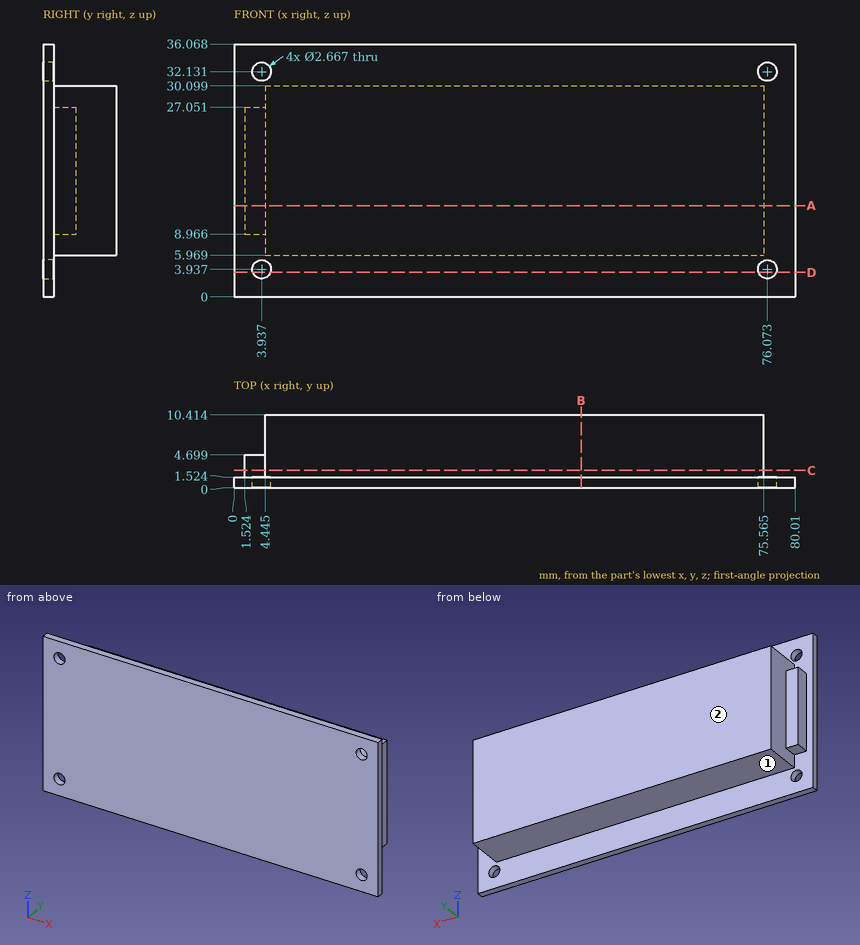
Here's the drawing with two shaded views (mm, measured from the low corner). I have some questions. A direction names the side the tool comes from. Coordinates: 2 decimals unless noted, no trailing zeros. Order: outer loops, then holes, each group sorted by start corner. A loop starts at its lowest first (then second) coordinate and runs counter-clockwise, first axis right, second up. Notation, with made-up numbers: (26, 35.25) - (76, 35.25) arc R17 ccw to (76, 50.25) - close; hole circle Ø8 at (-25.75, -32). An arc over 180 degrees is marked (long way). Answer in a Markdown table with one row per item. Add a question column.
(1) If we section it at B-B, the plane x = 49.5: Please give me the cut outline in (y, z).
(2) If we section it at A-A, the plane z = 13: Please give me the cut outline in (x, y) (3 decimals).
(3) If we section it at C-C, the plane y = 2.5: Please give me the cut outline in (x, z) (1 decimal), then the cut area to 3 significant figures.
(4) On a 3-axis mill with a long thin cutter (end or side, diameter ignored), from which of +Z, -Z, +X, -X, +Y, -Y can I reach the whole of each face in a straight line? I mean the marked faces 1 and 2. Say none if no direction works.
(5) If we section it at D-D, the plane z = 3.5: Please give me the cut outline in (x, y).
(6) Will these pins go through, and if not, where does the flat tip stop? pin 1 (3 mm diameter, centred on x = 26.5, y = 3.5, fed in from -Z); pin 2 (1.6 mm diameter, centred on y = 4, z = 16.5, fed in from -X); pin 3 (2.5 mm diameter, centred on x = 2.5, y = 4, fed in from -Z).
(7) I need wall thicknesses on L1, parallel to Y at x = 8, z = 35.5; L2, parallel to Z at x = 27.5, y = 4.5; L3, parallel to X at y = 6, z = 18.5 (3 decimals). Which ranges of each line are inside material? Lowest first, please.
Results are:
| question | item | result |
|---|---|---|
| 1 | outline | (0, 0) - (1.52, 0) - (1.52, 5.97) - (10.41, 5.97) - (10.41, 30.1) - (1.52, 30.1) - (1.52, 36.07) - (0, 36.07) - close |
| 2 | outline | (0, 0) - (80.01, 0) - (80.01, 1.524) - (75.565, 1.524) - (75.565, 10.414) - (4.445, 10.414) - (4.445, 4.699) - (1.524, 4.699) - (1.524, 1.524) - (0, 1.524) - close |
| 3 | outline | (1.5, 9) - (4.4, 9) - (4.4, 6) - (75.6, 6) - (75.6, 30.1) - (4.4, 30.1) - (4.4, 27.1) - (1.5, 27.1) - close |
| 3 | area | 1,770 mm2 |
| 4 | face 1 | -Z, +X, -X, +Y |
| 4 | face 2 | +Z, -Z, +X, -X, +Y |
| 5 | outline | (0, 0) - (2.68, 0) - (2.68, 1.52) - (0, 1.52) - close; (5.2, 0) - (74.81, 0) - (74.81, 1.52) - (5.2, 1.52) - close; (77.33, 0) - (80.01, 0) - (80.01, 1.52) - (77.33, 1.52) - close |
| 6 | pin 1 | stops at z = 5.97 |
| 6 | pin 2 | stops at x = 1.52 |
| 6 | pin 3 | stops at z = 8.97 |
| 7 | L1 | y = 0 to 1.52 |
| 7 | L2 | z = 5.97 to 30.1 |
| 7 | L3 | x = 4.445 to 75.565 |
